The listing builds one solid part. Answer for the finished solid, in the listing's coordinates (mm). Face numbers are marked on the shaded views. A direction names the side the tool comes from. Round coordinates to 2 decimals unless told otherwise and drop trailing zeros. Write each loop counter-clockwise with the first axis right and the second up, starting at its lowest first coordinate (ties: lowest second). Pieces come first, ordered by that corner, then holes. Notation, with made-up numbers: (-15.75, -7) - (31.25, -7) arc R9 cw to (31.25, 6) - close; hole circle Ø5 at (53.25, 1). An arc over 180 degrees is marked (long way). Return JSON: item names as keys, results as strings. Group by question number.
(1) Section D-D, the plane x = -3.5 is taken. Write down the section's boundary in (y, z).
(2) Determine the mould class of the marked faces 3, 4, 5 and 6 for opening direction X: +X half, -X half, draft (parallel to the pull), parting line (faces both ways), or undercut.
(3) Section C-C, the plane y = -3 is taken. Write down the section's boundary in (x, z), then the cut area to 3 significant figures.
(4) Section A-A, the plane x = 0 is taken. Write down the section's boundary in (y, z), then the cut area to 3 significant figures.
(5) This flat-tipped pin is pushed along its axis until it touches: pin 1 (3 mm diameter, centred on x = -0.5, z = -1, fed in from +Y). Where does it stop, or does it pass through?
(6) Find the intervals of material crossed by line 1 along X through (y, z) = (-4.1, 0); line 2 along Z through (x, y) = (0.5, -4.2); line 3 along Y through (x, z) = (5, 4.5), in increasing order. Write a range as [from, to].
(7) Section B-B, the plane z = 0 is taken. Write down the section's boundary in (x, y).
(8) Which of the six approach directions +Z, -Z, +X, -X, +Y, -Y give full straight-line access (tool end or side, diameter ignored) to the marked faces 1 and 2?
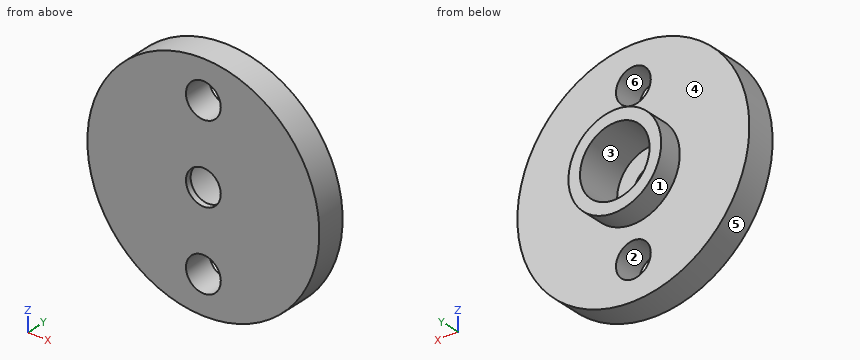
```python
from build123d import *

# Parameters (mm, degrees)
SKETCH4_R          = 1.5
CUT_EXTRUDE1_DEPTH = 15.361406616
CIRPATTERN1_COUNT  = 4


with BuildPart() as part:
    # Sketch1 → Revolve1 (revolve)
    with BuildSketch(Plane.XY, mode=Mode.PRIVATE) as revolve1_sk:
        Polygon((3, 0), (4, 0), (4, -2), (10, -2), (10, -4.5), (1.5, -4.5), (1.5, -4), (3, -4), align=None)
    revolve(revolve1_sk.sketch.rotate(Axis((0, 3.424478083, 0), (0, -1, 0)), 90), axis=Axis((0, 3.424478083, 0), (0, -1, 0)))

    # Sketch4 → Cut-Extrude1 (cut, through all)
    with BuildSketch(Plane(origin=(0, -2, 0), x_dir=(1, 0, 0), z_dir=(0, 1, 0))):
        with Locations(Location((0, 6.75, 0), (0, 0, 270))):
            Circle(SKETCH4_R)
    cut_extrude1 = extrude(amount=-CUT_EXTRUDE1_DEPTH, mode=Mode.SUBTRACT)

    # CirPattern1: Cut-Extrude1 ×4 about axis
    cirpattern1_axis = Axis((-7.809580464, -4.5, 0), (1, 0, 0))
    for i in range(1, CIRPATTERN1_COUNT):
        add(cut_extrude1.rotate(cirpattern1_axis, i * 360 / CIRPATTERN1_COUNT), mode=Mode.SUBTRACT)


solid = part.part
```
Working result:
{
 "1": {"outline": "(-4.5, -9.37) - (-2, -9.37) - (-2, -1.94) - (0, -1.94) - (0, 1.94) - (-2, 1.94) - (-2, 9.37) - (-4.5, 9.37) - close"},
 "2": {"face 3": "undercut", "face 4": "draft", "face 5": "parting line", "face 6": "undercut"},
 "3": {"outline": "circle Ø20 at (0, 0); hole circle Ø6 at (0, 0); hole circle Ø3 at (0, -6.75); hole circle Ø3 at (0, 6.75)", "area": "272 mm^2"},
 "4": {"outline": "(-4.5, -10) - (-2, -10) - (-2, -8.25) - (-4.5, -8.25) - close; (-4.5, -5.25) - (-2, -5.25) - (-2, -4) - (0, -4) - (0, -3) - (-4, -3) - (-4, -1.5) - (-4.5, -1.5) - close; (-4.5, 1.5) - (-4, 1.5) - (-4, 3) - (0, 3) - (0, 4) - (-2, 4) - (-2, 5.25) - (-4.5, 5.25) - close; (-4.5, 8.25) - (-2, 8.25) - (-2, 10) - (-4.5, 10) - close", "area": "25.5 mm^2"},
 "5": {"pin 1": "stops at y = -4"},
 "6": {"line 1": "x = [-10, -1.5], [1.5, 10]", "line 2": "z = [-9.99, -8.16], [-5.34, -1.41], [1.41, 5.34], [8.16, 9.99]", "line 3": "y = [-4.5, -2]"},
 "7": {"outline": "(-10, -4.5) - (-1.5, -4.5) - (-1.5, -4) - (-3, -4) - (-3, 0) - (-4, 0) - (-4, -2) - (-10, -2) - close; (1.5, -4.5) - (10, -4.5) - (10, -2) - (4, -2) - (4, 0) - (3, 0) - (3, -4) - (1.5, -4) - close"},
 "8": {"face 1": "+Y", "face 2": "+Y, -Y"}
}
